Here's the drawing with two shaded views (mm, measured from the low corner). I have some questions. Round coordinates to 2 decimals unless told otherwise and drop trailing zeros. Write each loop counter-clockwise with the first axis right and the second up, starting at its lowest first coordinate (ties: lowest second). Pieces come first, ordered by that corner, then holes.
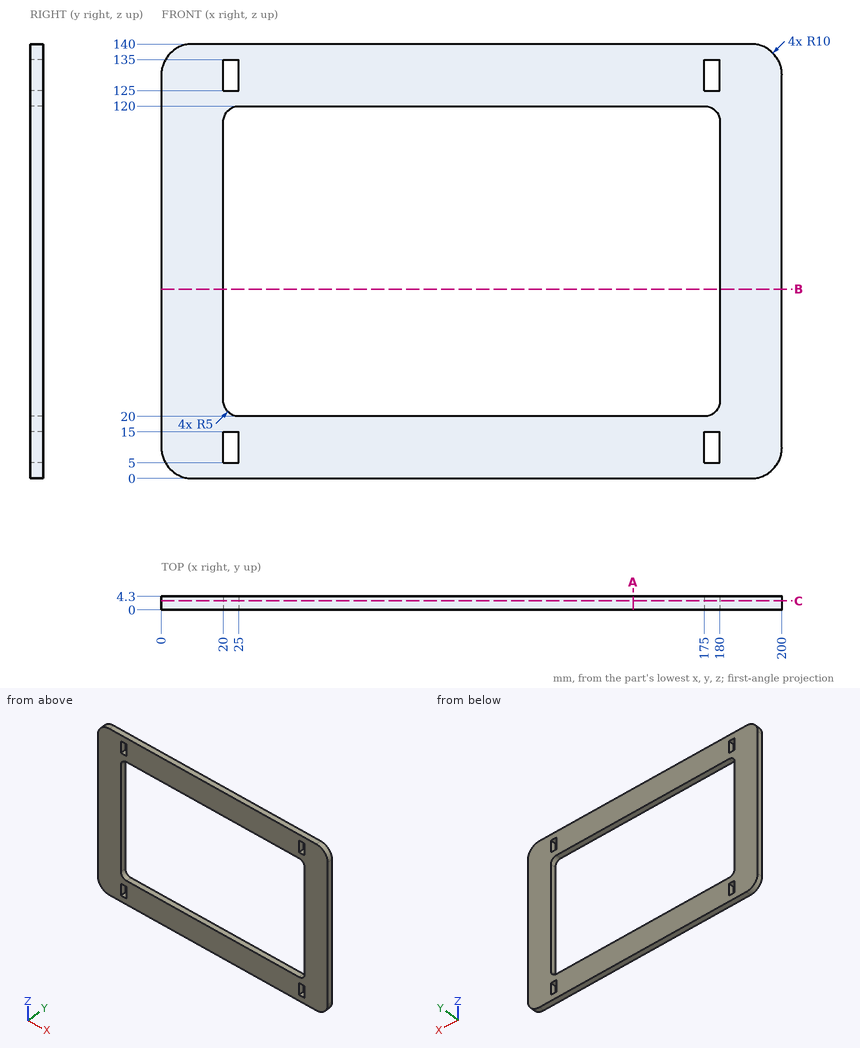
Q1. If I drill on L1, parallel to Z at x = 106.5, y = 0.9; L2, parallel to X at y = 0.95, z = 66.5; L3, parallel to X at y = 1.1, z = 6, over which ranges is the centre line in solid material (lowest first)?
Q2. Imagine slicing it at B-B, the plane z = 61. Write out the boundary of the cut face in (x, y), then the cut area to 3 significant figures.
Q3. I'm going to push flat-ended pins straight in: pin 1 Ø1.3 at (y, z) = (1, 8) entering from -X; pin 2 Ø1.3 at (y, z) = (2.5, 132) entering from +X. Where does each tip first touch, or does it pass through?
Q4. Imagine slicing it at C-C, the plane y = 2.9. Count the separate pieces of the cut face and the enclosed holes in it, then the cut area to 3 significant figures.
Q5. Imagine slicing it at A-A, the plane x = 152. Write out the boundary of the cut face in (y, z), then the cut area to 3 significant figures.
Results found:
1. L1: z = 0 to 20, 120 to 140
1. L2: x = 0 to 20, 180 to 200
1. L3: x = 0.83 to 20, 25 to 175, 180 to 199.17
2. outline: (0, 0) - (20, 0) - (20, 4.3) - (0, 4.3) - close; (180, 0) - (200, 0) - (200, 4.3) - (180, 4.3) - close
2. area: 172 mm2
3. pin 1: stops at x = 0.09
3. pin 2: stops at x = 199.91
4. separate pieces: 1
4. enclosed holes: 5
4. area: 11,700 mm2
5. outline: (0, 0) - (4.3, 0) - (4.3, 20) - (0, 20) - close; (0, 120) - (4.3, 120) - (4.3, 140) - (0, 140) - close
5. area: 172 mm2
